Source: CAD feature listing. Evaluate the final solid. Frame: model axes, mm. A direction names the side the tool comes from. Round coordinates to 2 decimals unless told otherwise and drop trailing zeros. Order: outer loops, then holes, each group sorted by start corner. A loop starts at its lowest first (then second) coordinate and runs counter-clockwise, first axis right, second up. Notation, with made-up numbers: (-4, -6) - (15, -6) arc R30 cw to (15, 20) - close; hole circle Ø8 at (87.25, 61). An arc over 180 degrees is marked (long way). Return JSON: item names as keys, results as strings. Group by question number.
1) Access query for faces 4 (the flat face through (0, 0, 46.5)), 5 (the flat face through (0, -5, 52.5)). Directions: +Z, -Z, +X, -X, +Y, -Y. A direction counts if a zero-diameter tool reaches every point of the face in a straight line with its end or side. Return the directions, or none.
2) Section A-A, the plane x = 0. Return loops of the section in (y, z), plus the area to 3 significant figures.
3) Contact query for flat-ended pins moving along their axis: P1, Ø1.5, axis at x = 7, z = 31.5, coming from the -Y side; P2, Ø2, axis at x = 2, z = 45, coming from the -Y side; P3, Ø2, axis at x = -8.5, z = 30, coming from the +Y side. Output: stop coordinate, or through.
4) Ray query, line 1 (Z direction, x = 4, y = 3); line 2 (X direction, y = 5, z = 43); line 3 (X direction, y = -10, z = 45.5). Return the intervals inside material, ascending. Write a range as from..to.
5) Mould query, pull axis Y, two halves, no side actions, for faces 1 (the cylindrical face through (-0.39, -1.77, 49.46)), 2 (the flat face through (0, 4, 52.5)), 3 (the cylindrical face through (1.5, -11.4, 22.9)). Classes: pulls with the +Y half, pulls with the -Y half, needs draft (parallel to the pull), parting line crosses it, or undercut.
6) Section B-B, the plane z = 7.5. Return loops of the section in (x, y).
```python
from build123d import *

# Parameters (mm, degrees)
SKETCH1_R           = 11.5
BOSS_EXTRUDE1_DEPTH = 46.5
FILLET1_R           = 1
SKETCH2_R           = 3
BOSS_EXTRUDE2_DEPTH = 6


with BuildPart() as part:
    # Sketch1 → Boss-Extrude1 (new body)
    with BuildSketch(Plane.XY):
        with Locations(Location((0, 0, 0), (0, 0, 180))):
            Circle(SKETCH1_R)
    extrude(amount=BOSS_EXTRUDE1_DEPTH)

    # Fillet1
    fillet1_edges = [part.edges().sort_by_distance(p)[0] for p in [
        (11.5, 0, 0),
        (11.5, 0, 46.5),
    ]]
    fillet(fillet1_edges, radius=FILLET1_R)

    # Sketch2 → Boss-Extrude2 (add)
    with BuildSketch(Plane.XY.offset(46.5)):
        with Locations((0, -4.744469282)):
            Circle(SKETCH2_R)
        with Locations((0, 4.441817119)):
            Circle(SKETCH2_R)
    extrude(amount=BOSS_EXTRUDE2_DEPTH)


solid = part.part
```
Geometry check:
{
 "1": {"face 4": "+Z", "face 5": "+Z, +X, -X, +Y, -Y"},
 "2": {"outline": "(-11.5, 1) arc R1 ccw to (-10.5, 0) - (10.5, 0) arc R1 ccw to (11.5, 1) - (11.5, 45.5) arc R1 ccw to (10.5, 46.5) - (7.44, 46.5) - (7.44, 52.5) - (1.44, 52.5) - (1.44, 46.5) - (-1.74, 46.5) - (-1.74, 52.5) - (-7.74, 52.5) - (-7.74, 46.5) - (-10.5, 46.5) arc R1 ccw to (-11.5, 45.5) - close", "area": "1,140 mm2"},
 "3": {"P1": "y = -9.65", "P2": "y = -11.46", "P3": "y = 8.72"},
 "4": {"line 1": "0..46.5", "line 2": "-10.36..10.36", "line 3": "-5.68..5.68"},
 "5": {"face 1": "undercut", "face 2": "needs draft", "face 3": "parting line crosses it"},
 "6": {"outline": "circle Ø23 at (0, 0)"}
}
